Can you work these out from the drawing? Everything is in mm from the part's minimum corner. Coordinates: 2 decimals unless noted, no trailing zeros. Loops run counter-clockwise (first coordinate to the right, second up) from the corner with the lowest first, then second, coordinate; pieces in that order, holes last. Notation, with made-up numbers: (-0.5, 64) - (41.5, 64) arc R16 cw to (41.5, 71) - close; hole circle Ø4 at (32, 15.25). An arc over 180 degrees is marked (long way). One line per question, with ' | ' between items. Start each with the question number.
1. I want a section at C-C, the plane y = 99. Write out the boundary of the cut face in (x, z), then the cut area to 3 significant figures.
2. I want a section at A-A, the plane z = 10.5. Write out the boundary of the cut face in (x, y), then the cut area to 3 significant figures.
3. I want a section at B-B, the plane x = 10.5. Write out the boundary of the cut face in (y, z), then the cut area to 3 significant figures.
4. Please list where these lines run through material, in increasing order: L1, parallel to Y at x = 16.25, z = 10.5; L2, parallel to Y at x = 11.25, z = 13.5; L3, parallel to Z at x = 1.5, y = 16. Write a range as [from, to].
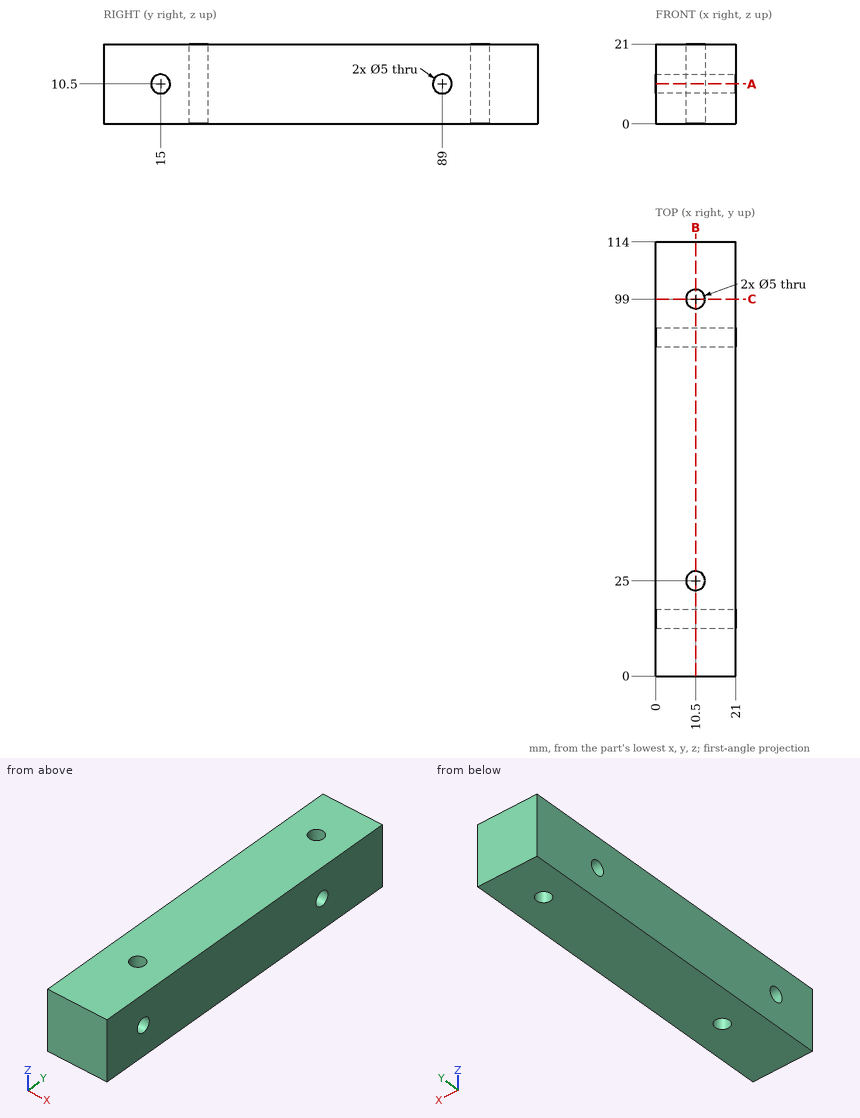
Results are:
1) outline: (0, 0) - (8, 0) - (8, 21) - (0, 21) - close; (13, 0) - (21, 0) - (21, 21) - (13, 21) - close | area: 336 mm2
2) outline: (0, 0) - (21, 0) - (21, 12.5) - (0, 12.5) - close; (0, 17.5) - (21, 17.5) - (21, 86.5) - (0, 86.5) - close; (0, 91.5) - (21, 91.5) - (21, 114) - (0, 114) - close; hole circle Ø5 at (10.5, 25); hole circle Ø5 at (10.5, 99) | area: 2,140 mm2
3) outline: (0, 0) - (22.5, 0) - (22.5, 21) - (0, 21) - close; (27.5, 0) - (96.5, 0) - (96.5, 21) - (27.5, 21) - close; (101.5, 0) - (114, 0) - (114, 21) - (101.5, 21) - close; hole circle Ø5 at (15, 10.5); hole circle Ø5 at (89, 10.5) | area: 2,140 mm2
4) L1: y = [0, 12.5], [17.5, 86.5], [91.5, 114] | L2: y = [0, 22.62], [27.38, 96.62], [101.38, 114] | L3: z = [0, 8.21], [12.79, 21]
